Input: dimensioned drawing with shaded views. Units: mm. Origin: part minimum x, y, z. A direction names the side the tool comes from. Round coordinates to 2 decimals unless told otherwise and drop trailing zeros. Order: outer loops, then holes, each group sorted by start corner. A loop starts at its lowest first (then second) coordinate and runs counter-clockwise, first axis right, second up. Notation, with made-up numbers: M -34,49 L -20,49 A13 ccw -20,68 Z; hole C -5,-26.75 d10. An arc over 180 degrees is marked long. Use one line per item in the form item = value. Start each with the question number.
Q1. Section A-A (z = 7). Return the cut outline in (x, y) (1 decimal).
Q2. Section D-D (x = 49). Return the cut outline in (y, z), plus the area to 3 significant figures.
Q3. Section B-B (x = 59). Return the cut outline in (y, z).
Q4. Contact query for flat-ended pins moving along their axis: pin 1 (6 mm diameter, centred on x = 49, z = 24.5, fed in from +Y) (1 decimal); pin 2 (1 mm diameter, centred on x = 14.5, z = 52, fed in from -Y) (1 decimal); pin 3 (6 mm diameter, centred on x = 9.5, z = 6, fed in from +Y). Output: stop coordinate, or through.
Q5. Reachability of the marked faces 1, 2 and 3 from +Z, -Z, +X, -X, +Y, -Y: full face, straight path, thin tool, end or side. Return the list, or none.
Q6. Material intervals for probe 1 along Y at (x, z) = (50, 3.5) (1 decimal); probe 2 along X at (y, z) = (43, 12.25); probe 3 along Y at (x, z) = (46, 10) (1 decimal), sorted ascending.
Q7. Pull-direction query (Y, two-part tool) for the marked faces 4, 5, 6 and 7; classes: pulls with the +Y half, pulls with the -Y half, needs draft (parallel to the pull), parting line crosses it, or undercut.
Q8. Section C-C (y = 76). Return the cut outline in (x, z).
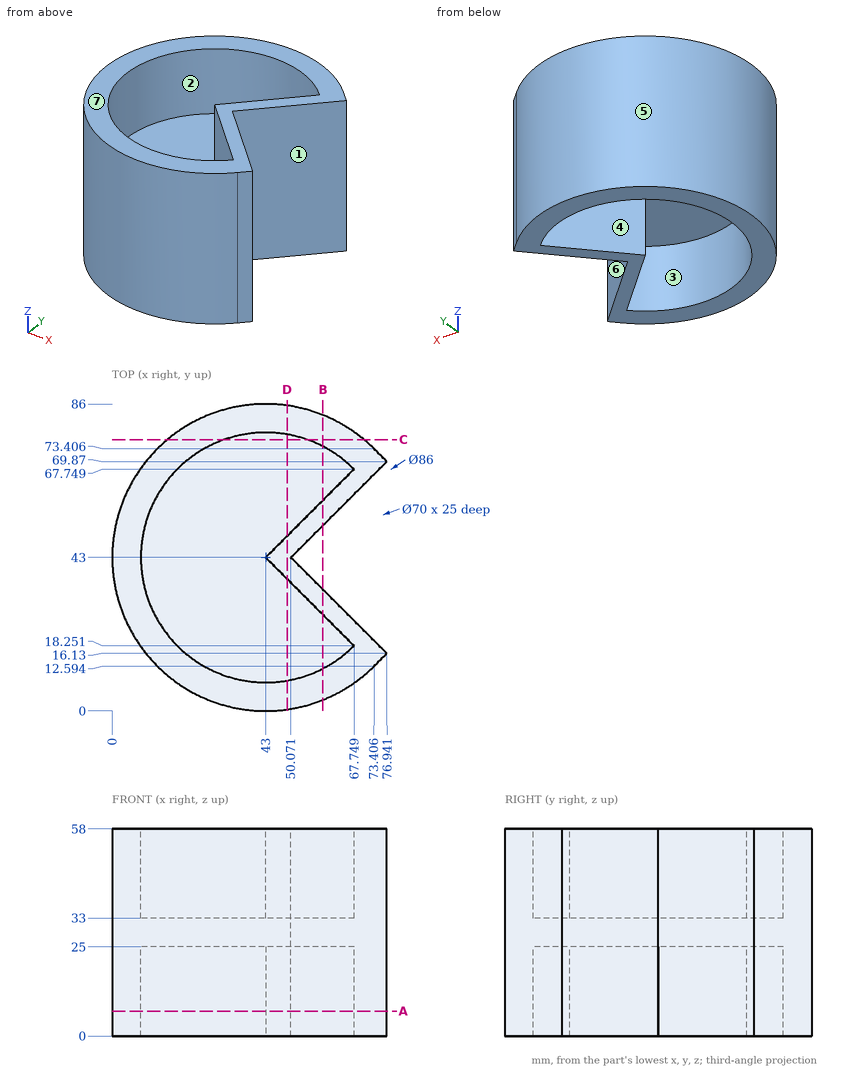
Results list:
q1.outline = M 50.1,43 L 76.9,69.9 L 73.4,73.4 A43 ccw long 73.4,12.6 L 76.9,16.1 Z; hole M 43,43 L 67.7,67.7 A35 ccw long 67.7,18.3 Z
q2.outline = M 0.42,0 L 8.52,0 L 8.52,25 L 37,25 L 37,0 L 49,0 L 49,25 L 77.48,25 L 77.48,0 L 85.58,0 L 85.58,58 L 77.48,58 L 77.48,33 L 49,33 L 49,58 L 37,58 L 37,33 L 8.52,33 L 8.52,58 L 0.42,58 Z
q2.area = 2,090 mm2
q3.outline = M 3.09,0 L 11.87,0 L 11.87,25 L 27,25 L 27,0 L 34.07,0 L 34.07,58 L 27,58 L 27,33 L 11.87,33 L 11.87,58 L 3.09,58 Z; M 51.93,0 L 59,0 L 59,25 L 74.13,25 L 74.13,0 L 82.91,0 L 82.91,58 L 74.13,58 L 74.13,33 L 59,33 L 59,58 L 51.93,58 Z
q4.pin_1 = 85.9
q4.pin_2 = 10.4
q4.pin_3 = 73.31
q5.face_1 = +Z, -Z, +X
q5.face_2 = +Z
q5.face_3 = -Z
q6.probe_1 = 0.6 to 8.7, 36 to 50, 77.3 to 85.4
q6.probe_2 = 0 to 8, 43 to 50.07
q6.probe_3 = 0.1 to 8.1, 40 to 46, 77.9 to 85.9
q7.face_4 = undercut
q7.face_5 = parting line crosses it
q7.face_6 = undercut
q7.face_7 = needs draft
q8.outline = M 15.43,0 L 31.34,0 L 31.34,25 L 54.66,25 L 54.66,0 L 70.57,0 L 70.57,58 L 54.66,58 L 54.66,33 L 31.34,33 L 31.34,58 L 15.43,58 Z
